Geometry: final body of the model. Coordinates: model frame, mm. A direction names the side the tool comes from. Coordinates: 2 decimals unless noted, no trailing zeros. Order: outer loops, then holes, each group sorted by start corner. A loop starts at its lowest first (then second) coordinate and runs counter-clockwise, first axis right, second up. Notation, with made-up numbers: M 85.5,-17.5 L 100.5,-17.5 A22 cw 100.5,-5.5 Z; hole C 63,-25.75 d11. An arc over 180 degrees is marked long. Use CSV: the item, a comma, the result in double quotes. Start each with the question number.
1. Material intervals for line 1 (Y direction, x = 8, z = 7); line 2 (Y direction, x = 1.5, z = 9); line 3 (X direction, y = 17, z = 9), sorted ascending.
2. First-contact query: P1, Ø5, axis at y = -19.5, z = 9, coming from the +X side. Flat tip, straight axial feed; report the tip coordinate or a pass-through.
3. Section query B-B on z = 7. Return the cut outline in (x, y).
4. Section query C-C on x = -16. Return the cut outline in (y, z), and give its area (3 significant figures).
5. Section query A-A on y = 37.5. Return the cut outline in (x, z), and give its area (3 significant figures).
6. Pull-direction query (Y, two-part tool) for faces 1 (the cylindrical face through (-0.3, -48.43, 9.4)), 2 (the flat face through (0, 41, 5)), 3 (the flat face through (0, 1, 10)); classes: pulls with the +Y half, pulls with the -Y half, needs draft (parallel to the pull), parting line crosses it, or undercut.
7. Set-up query: faces 4 (the flat face through (0, 34, 5)), 5 (the flat face through (0, -49, 4)). Return all of +Z, -Z, +X, -X, +Y, -Y with unobstructed straight access to the full face (end or side cutting, diameter ignored); none if empty.
from build123d import *

# Parameters (mm, degrees)
PAD_DEPTH = 10
FILLET_R  = 2


with BuildPart() as part:
    # Sketch → Pad (new body)
    with BuildSketch(Plane.XY):
        with BuildLine():
            Line((-21.5, 49), (21.5, 49))
            ThreePointArc((25, 45.5), (23.974874, 47.974874), (21.5, 49))
            Line((25, 45.5), (25, -45.5))
            ThreePointArc((21.5, -49), (23.974874, -47.974874), (25, -45.5))
            Line((21.5, -49), (-21.5, -49))
            ThreePointArc((-25, -45.5), (-23.974874, -47.974874), (-21.5, -49))
            Line((-25, -45.5), (-25, 45.5))
            ThreePointArc((-21.5, 49), (-23.974874, 47.974874), (-25, 45.5))
        make_face()
        with BuildLine():
            ThreePointArc((-13.5, 41), (-17, 37.5), (-13.5, 34))
            Line((-13.5, 34), (13.5, 34))
            ThreePointArc((13.5, 34), (17, 37.5), (13.5, 41))
            Line((13.5, 41), (-13.5, 41))
        make_face(mode=Mode.SUBTRACT)
        with BuildLine():
            ThreePointArc((-13.5, -34), (-17, -37.5), (-13.5, -41))
            Line((-13.5, -41), (13.5, -41))
            ThreePointArc((13.5, -41), (17, -37.5), (13.5, -34))
            Line((13.5, -34), (-13.5, -34))
        make_face(mode=Mode.SUBTRACT)
    extrude(amount=PAD_DEPTH)

    # Fillet
    fillet_edges = [part.edges().sort_by_distance(p)[0] for p in [
        (-25, 0, 10),
    ]]
    fillet(fillet_edges, radius=FILLET_R)


solid = part.part
Results list:
1,line 1,"y = -49 to -41, -34 to 34, 41 to 49"
1,line 2,"y = -48.73 to -41, -34 to 34, 41 to 48.73"
1,line 3,"x = -24.73 to 24.73"
2,P1,"stops at x = 25"
3,outline,"M -25,-45.5 A3.5 ccw -21.5,-49 L 21.5,-49 A3.5 ccw 25,-45.5 L 25,45.5 A3.5 ccw 21.5,49 L -21.5,49 A3.5 ccw -25,45.5 Z; hole M -13.5,-41 L 13.5,-41 A3.5 ccw 13.5,-34 L -13.5,-34 A3.5 ccw Z; hole M -13.5,34 L 13.5,34 A3.5 ccw 13.5,41 L -13.5,41 A3.5 ccw Z"
4,outline,"M -49,0 L -39.95,0 L -39.95,10 L -47,10 A2 ccw -49,8 Z; M -35.05,0 L 35.05,0 L 35.05,10 L -35.05,10 Z; M 39.95,0 L 49,0 L 49,8 A2 ccw 47,10 L 39.95,10 Z"
4,area,"880 mm²"
5,outline,"M -25,0 L -17,0 L -17,10 L -23,10 A2 ccw -25,8 Z; M 17,0 L 25,0 L 25,8 A2 ccw 23,10 L 17,10 Z"
5,area,"158 mm²"
6,face 1,"pulls with the -Y half"
6,face 2,"undercut"
6,face 3,"needs draft"
7,face 4,"+Z, -Z"
7,face 5,"+Z, -Z, +X, -X, -Y"
